Autodesk Fusion 360 part; units mm, degrees
sketch "Sketch1" plane through (0, 0, 0) normal (0, 0, 1) x (1, 0, 0)
  line L0 (50, 30) -> (-50, 30)
  line L1 (-50, 30) -> (-50, -30)
  line L2 (-50, -30) -> (50, -30)
  line L3 (50, -30) -> (50, 30)
  line L4 (50, 30) -> (-50, -30) construction
  line L5 (-50, 30) -> (50, -30) construction
  line L6 (-50, 30) -> (-25, 30)
  line L7 (-25, 30) -> (-25, 10)
  line L8 (-25, 10) -> (-50, 10)
  line L9 (-50, 10) -> (-50, 30)
  line L10 (-25, 30) -> (25, 30)
  line L11 (25, 30) -> (25, 10)
  line L12 (25, 10) -> (-25, 10)
  line L13 (-25, 10) -> (-25, 30)
  line L14 (25, 30) -> (50, 30)
  line L15 (50, 30) -> (50, 10)
  line L16 (50, 10) -> (25, 10)
  line L17 (25, 10) -> (25, 30)
  dimension "d1" = 100
  dimension "d2" = 60
  dimension "d3" = 25
  dimension "d4" = 50
  dimension "d5" = 20
extrude "Extrude1" add sketch "Sketch1" along normal blind 20 contours L1 L2 L3 L8 L12 L16
extrude "Extrude2" add sketch "Sketch1" along normal blind 45 contours L0 L3 L11 L14 L15 L16 L17 | L0 L7 L10 L11 L12 L13 L17 | L0 L1 L6 L7 L8 L9 L13
sketch "Sketch2" plane through (0, 0, 0) normal (0, 1, 0) x (1, 0, 0)
sketch "Sketch3" plane through (0, 10, 0) normal (0, -1, 0) x (1, 0, 0)
  line L0 (-50, 20) -> (50, 20)
  line L1 (50, 20) -> (50, 45)
  line L2 (-50, 45) -> (-50, 20)
  circle A0 centre (0, 45) radius 20
  arc A1 (25, 45) -> (-25, 45) centre (0, 45) ccw
  line L3 (-25, 45) -> (-20, 45)
  line L4 (20, 45) -> (25, 45)
  dimension "d10" = 40
hole "Hole1" at (0, 10, 45) direction (0, 1, 0) diameter 40 depth 40 tip angle 118
extrude "Extrude3" add sketch "Sketch3" against normal blind 20 contours A0 A1 L3 L4
sketch "Sketch4" plane through (50, 0, 0) normal (1, 0, 0) x (0, 1, 0)
  line L0 (-30, 0) -> (30, 0)
  line L1 (30, 0) -> (30, 45)
  line L2 (30, 45) -> (10, 45)
  line L3 (10, 45) -> (10, 20)
  line L4 (10, 20) -> (-30, 20)
  line L5 (-30, 20) -> (-30, 0)
The listing builds one solid part. Answer for the finished solid, in the listing's coordinates (mm). A direction names the side the tool comes from. Give positions to 0.01 mm unless a question says otherwise; leave off trailing zeros. Write each loop counter-clockwise with the first axis right and the second up, starting at its lowest first coordinate (ties: lowest second). Pieces come first, ordered by that corner, then holes. Notation, with made-up numbers: M -13.75,88 L 7.25,88 A22 ccw 7.25,110 Z; hole C 6,14.25 d2. An arc over 180 degrees is marked long. Write each question's results on one line, items separated by ' | '.
Q1. Section C-C, the plane y = 14.5 is taken. Write down the section's boundary in (x, z), then the cut area to 3 significant figures.
Output values:
outline: M -50,0 L 50,0 L 50,45 L 25,45 A25 ccw -25,45 L -50,45 Z; hole C 0,45 d40 | area: 4,230 mm2
Q2. A tool of negligible diameter and unlimited length cuts with its end or side. For faces 1 (the cylindrical face through (0.55, 19.86, 69.994)), 2 (the flat face through (-1, -10, 20)), 3 (the flat face through (-38, 20, 45)), 4 (the flat face through (-50, 7, 17)), 5 (the flat face through (37, 20, 45)), from which of +Z, -Z, +X, -X, +Y, -Y can it reach the whole face along a straight path? Write none if from no direction.
Output values:
face 1: +Z, +Y, -Y | face 2: +Z, +X, -X, -Y | face 3: +Z, -X, +Y, -Y | face 4: +Z, -Z, -X, +Y, -Y | face 5: +Z, +X, +Y, -Y
Q3. Section B-B, the plane z = 42.5 is taken. Write down the section's boundary in (x, y).
Output values:
outline: M -50,10 L -19.84,10 L -19.84,30 L -50,30 Z; M 19.84,10 L 50,10 L 50,30 L 19.84,30 Z
Q4. Consider L1, parallel to Z at x = -0.5, y = 22 (3 decimals); L2, parallel to Z at x = -45, y = -6; L3, parallel to Y at x = 18, z = 24.5. Determine where each line is inside the solid, lowest interval first. Write a range as from..to.
Output values:
L1: 0..25.006, 64.994..69.995 | L2: 0..20 | L3: 10..30
Q5. Flat-ended cylindrical pins translate along their axes: P1, Ø10, axis at x = 5, z = 26.5, coming from the -Y side; P2, Ø12, axis at x = -9, z = 28.5, coming from the +Y side; P3, Ø4, axis at x = -28, y = 11.5, coming from the +Z side; P4, Ø2, axis at x = -14.5, y = 18.5, coming from the +Z side. Find the tip coordinate at first contact, or state that the pin passes through.
Output values:
P1: y = 10 | P2: y = 30 | P3: z = 45 | P4: z = 66.04
Q6. Section D-D, the plane x = -27 is taken. Write down the section's boundary in (y, z).
Output values:
outline: M -30,0 L 30,0 L 30,45 L 10,45 L 10,20 L -30,20 Z
Q7. Section A-A, the plane x = 0 is taken. Write down the section's boundary in (y, z), then the cut area to 3 significant figures.
Output values:
outline: M -30,0 L 30,0 L 30,25 L 10,25 L 10,20 L -30,20 Z; M 10,65 L 30,65 L 30,70 L 10,70 Z | area: 1,400 mm2
